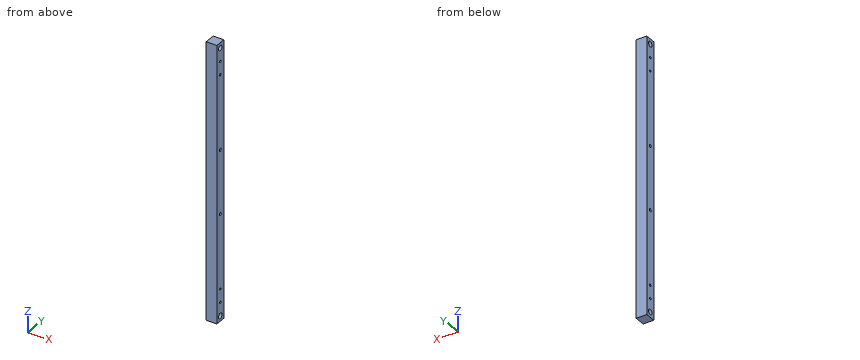
```python
from build123d import *

# Parameters (mm, degrees)
SKETCH1_W               = 25.4
SKETCH1_H               = 25.4
BOSS_EXTRUDE1_DEPTH     = 660.4
SKETCH2_R               = 6.35
CUT_EXTRUDE4_DEPTH      = 26.4
CUT_EXTRUDE4_DEPTH_BACK = 1
SKETCH3_R               = 2.55
CUT_EXTRUDE5_DEPTH      = 26.4
SKETCH10_R              = 3.5
CUT_EXTRUDE6_DEPTH      = 26.4


with BuildPart() as part:
    # Sketch1 → Boss-Extrude1 (new body)
    with BuildSketch(Plane.XY):
        Rectangle(SKETCH1_W, SKETCH1_H)
    extrude(amount=BOSS_EXTRUDE1_DEPTH)

    # Sketch2 → Cut-Extrude4 (cut, two sides)
    with BuildSketch(Plane(origin=(-12.7, 0, 0), x_dir=(0, 0, -1), z_dir=(1, 0, 0))) as cut_extrude4_sk:
        with Locations((-12.7, 0)):
            Circle(SKETCH2_R)
        with Locations((-647.7, 0)):
            Circle(SKETCH2_R)
    extrude(amount=CUT_EXTRUDE4_DEPTH, mode=Mode.SUBTRACT)
    extrude(cut_extrude4_sk.sketch, amount=-CUT_EXTRUDE4_DEPTH_BACK, mode=Mode.SUBTRACT)

    # Sketch3 → Cut-Extrude5 (cut, through all)
    with BuildSketch(Plane.ZY.offset(12.7)):
        with Locations((584.2, 0)):
            Circle(SKETCH3_R)
        with Locations((76.2, 0)):
            Circle(SKETCH3_R)
        with Locations((615.95, 0)):
            Circle(SKETCH3_R)
        with Locations((44.45, 0)):
            Circle(SKETCH3_R)
    extrude(amount=-CUT_EXTRUDE5_DEPTH, mode=Mode.SUBTRACT)

    # Sketch10 → Cut-Extrude6 (cut, through all)
    with BuildSketch(Plane.ZY.offset(12.7)):
        with Locations((406.4, 0)):
            Circle(SKETCH10_R)
        with Locations((254, 0)):
            Circle(SKETCH10_R)
    extrude(amount=-CUT_EXTRUDE6_DEPTH, mode=Mode.SUBTRACT)


solid = part.part
```
Read the model definition and answer for the solid it produces. Units are mm, in the model's axes. Round coordinates to 2 decimals unless told otherwise and drop trailing zeros. Write each loop counter-clockwise with the first axis right and the second up, starting at its lowest first coordinate (ties: lowest second). Pieces come first, ordered by that corner, then holes. Notation, with made-up numbers: (-19.75, -20) -> (19.25, -20) arc R22 ccw to (19.25, 4) -> close; hole circle Ø5 at (63, 83.5). An arc over 180 degrees is marked (long way). Answer in a Markdown table with one row per item. Add a question column.
1) Find section A-A, the plane z = 12.7. Determine the outline of the cut face in (x, y).
2) Given P1, Ø11, axis at y = 0, z = 406.4, coming from the +X side; P2, Ø11.5, axis at y = 0, z = 647.7, coming from the -X side, each flat-ended and moving along its own axis, determine where each tip first touches the part or whether it passes through.
3) Consider line 1 (Z direction, x = -5.75, y = -3.75); line 2 (Z direction, x = -6.25, y = 4.5); line 3 (Y direction, x = -2.75, z = 584.2). Determine where each line is inside the solid, lowest interval first.
4) Find section B-B, the plane x = 8.5. State how many separate pieces and enclosed holes the cut face has, and give its area (3 significant figures).
Findings below:
| question | item | result |
|---|---|---|
| 1 | outline | (-12.7, -12.7) -> (12.7, -12.7) -> (12.7, -6.35) -> (-12.7, -6.35) -> close; (-12.7, 6.35) -> (12.7, 6.35) -> (12.7, 12.7) -> (-12.7, 12.7) -> close |
| 2 | P1 | x = 12.7 |
| 2 | P2 | through |
| 3 | line 1 | 0 to 7.58, 17.82 to 642.58, 652.82 to 660.4 |
| 3 | line 2 | 0 to 8.22, 17.18 to 643.22, 652.18 to 660.4 |
| 3 | line 3 | -12.7 to -2.55, 2.55 to 12.7 |
| 4 | separate pieces | 1 |
| 4 | enclosed holes | 8 |
| 4 | area | 16,400 mm² |
